Can you work these out from the model? Positions are in its coordinate system, mm. A direction names the side the tool comes from. Round coordinates to 2 decimals unless told otherwise and drop trailing zeros. Loops run counter-clockwise (first coordinate to the right, second up) from the corner with the lowest first, then second, coordinate; pieces in that order, holes last.
from build123d import *

# Parameters (mm, degrees)
F1_DEPTH = 20
F3_R     = 1.49999
F2_R     = 2
F4_DEPTH = 3


# Not quite as in the source:
# - a fillet or chamfer is up to 0.001 mm smaller than in the source, because OpenCascade refuses the exact size


with BuildPart() as f1:
    # F0 (on Top) → F1 (new body)
    with BuildSketch(Plane.XY):
        Polygon((11, 11), (-19, 11), (-19, 8), (-8, 8), (-3.7573593129, 8), (8, 8), (8, -3.7573593129), (8, -8), (8, -24), (11, -24), align=None)
        Polygon((-3.7573593129, 8), (-8, 8), (8, -8), (8, -3.7573593129), align=None)
    extrude(amount=F1_DEPTH)

    # F3 (radius 1.5 in the source; OpenCascade refuses exactly that, so slightly less here)
    f3_edges = [f1.edges().sort_by_distance(p)[0] for p in [
        (-19, 8, 10),
        (-19, 11, 10),
        (-8, 8, 10),
        (8, -24, 10),
        (11, -24, 10),
        (8, -8, 10),
        (8, 8, 10),
        (11, 11, 10),
        (-3.757359, 8, 10),
        (8, -3.757359, 10),
    ]]
    fillet(f3_edges, radius=F3_R)

    # F2 (on face) → F4 (cut, through all)
    with BuildSketch(Plane.XZ.offset(-8)):
        with Locations((-13, 10)):
            Circle(F2_R)
    extrude(amount=-F4_DEPTH, mode=Mode.SUBTRACT)


solid = f1.part
(1) For faces 4 (the flat face through (3, 8, 10)), 5 (the flat face through (-13.1, 8, 7.6)), 6 (the cylindrical face through (10.55, 10.57, 10.14)), which set-ups out of +Z, -Z, +X, -X, +Y, -Y let a thin tool reach every point of the face, with its end or its side?
Worked answers:
face 4: +Z, -Z
face 5: +Z, -Z, -X, -Y
face 6: +Z, -Z, +X, +Y
(2) If we section it at A-A, the plane x = -13: List the corners of the cut face in (y, z) for me.
Worked answers:
outline: (8, 0) - (11, 0) - (11, 8) - (8, 8) - close; (8, 12) - (11, 12) - (11, 20) - (8, 20) - close
(3) If we section it at B-B, the plane z = 10: State how many separate pieces and enclosed holes the cut face has, then the cut area to 3 significant figures.
Worked answers:
separate pieces: 2
enclosed holes: 1
area: 237 mm2
(4) If we section it at D-D, the plane y = -15: List the corners of the cut face in (x, z) for me, then the cut area to 3 significant figures.
Worked answers:
outline: (8, 0) - (11, 0) - (11, 20) - (8, 20) - close
area: 60.0 mm2
(5) If I drill on line 1 (Z direction, x = -13, y = 9.55); line 2 (X direction, y = -16, z = 8.5); line 3 (Y direction, x = -1, z = 8), over which ranges is the centre line in solid material (lowest first)?
Worked answers:
line 1: z = 0 to 8, 12 to 20
line 2: x = 8 to 11
line 3: y = 1 to 5.24, 7.73 to 11
(6) Will these pins go through, and if not, where does the flat tip stop? P1, Ø7.5, axis at y = 4, z = 8.5, coming from the -X side; P2, Ø4.5, axis at x = -14, z = 13, coming from the -Y side; P3, Ø12, axis at x = 1, z = 12.5, coming from the -Y side.
Worked answers:
P1: stops at x = -7.79
P2: stops at y = 8
P3: stops at y = -7
(7) If we mould it in two halves opening along X, with no side actions, what happens to faces 1 (the cylindrical face through (-1.51, 7.1, 10.14)), 2 (the flat face through (3, 1, 20)), 3 (the flat face through (11, -7, 10))? For each: released by +X, released by -X, zero draft, split by the parting line, or undercut.
Worked answers:
face 1: undercut
face 2: zero draft
face 3: released by +X
